from build123d import *

# Parameters (mm, degrees)
BOSS_EXTRUDE1_DEPTH      = 52.5
BOSS_EXTRUDE1_DEPTH_BACK = 52.5
BOSS_EXTRUDE2_DEPTH      = 13
BOSS_EXTRUDE3_DEPTH      = 13
CUT_EXTRUDE1_DEPTH       = 65.5
CUT_EXTRUDE1_DEPTH_BACK  = 65.5
CUT_EXTRUDE2_DEPTH       = 29
CUT_EXTRUDE2_DEPTH_BACK  = 29
CUT_EXTRUDE3_DEPTH       = 29
CUT_EXTRUDE3_DEPTH_BACK  = 29
SKETCH7_R                = 2.6
CUT_EXTRUDE4_DEPTH       = 1
SKETCH8_R                = 2.6
CUT_EXTRUDE5_DEPTH       = 1
CUT_EXTRUDE6_START       = 1
SKETCH9_R                = 2.6
CUT_EXTRUDE6_DEPTH       = 1
CUT_EXTRUDE7_START       = 1
SKETCH10_R               = 2.6
CUT_EXTRUDE7_DEPTH       = 1
CUT_EXTRUDE8_DEPTH       = 35
CUT_EXTRUDE9_DEPTH       = 35


with BuildPart() as part:
    # Sketch1 → Boss-Extrude1 (new, two sides: drawn at the far end of the back side and taken through both)
    with BuildSketch(Plane(origin=(0, 0, 0), x_dir=(0, 0, -1), z_dir=(1, 0, 0)).offset(-BOSS_EXTRUDE1_DEPTH_BACK)):
        with BuildLine():
            Line((-30, 33), (-30, 27))
            Line((-30, 27), (-29.5, 26.5))
            Line((-29.5, 26.5), (-29.5, 2))
            ThreePointArc((-29.5, 2), (-28.914213562, 0.585786438), (-27.5, 0))
            Line((-27.5, 0), (27.5, 0))
            ThreePointArc((27.5, 0), (28.914213562, 0.585786438), (29.5, 2))
            Line((29.5, 2), (29.5, 26.5))
            Line((29.5, 26.5), (30, 27))
            Line((30, 27), (30, 33))
            Line((30, 33), (28, 35))
            Line((28, 35), (10, 35))
            Line((10, 35), (9.5, 34.5))
            Line((9.5, 34.5), (-9.5, 34.5))
            Line((-9.5, 34.5), (-10, 35))
            Line((-10, 35), (-28, 35))
            Line((-28, 35), (-30, 33))
        make_face()
    extrude(amount=BOSS_EXTRUDE1_DEPTH + BOSS_EXTRUDE1_DEPTH_BACK)

    # Sketch2 → Boss-Extrude2 (add)
    with BuildSketch(Plane(origin=(-65.5, 0, 0), x_dir=(0, 0, -1), z_dir=(1, 0, 0))):
        Polygon((-29, 2), (-27, 0), (27, 0), (29, 2), (29, 32.5), (27.5, 34), (-27.5, 34), (-29, 32.5), align=None)
    extrude(amount=BOSS_EXTRUDE2_DEPTH)

    # Sketch3 → Boss-Extrude3 (add)
    with BuildSketch(Plane(origin=(65.5, 0, 0), x_dir=(0, 0, -1), z_dir=(1, 0, 0))):
        Polygon((-29, 2), (-27, 0), (27, 0), (29, 2), (29, 32.5), (27.5, 34), (-27.5, 34), (-29, 32.5), align=None)
    extrude(amount=-BOSS_EXTRUDE3_DEPTH)

    # Sketch4 → Cut-Extrude1 (cut, two sides: drawn at the far end of the back side and taken through both)
    with BuildSketch(Plane(origin=(0, 0, 0), x_dir=(0, 0, -1), z_dir=(1, 0, 0)).offset(-CUT_EXTRUDE1_DEPTH_BACK)):
        with BuildLine():
            Line((-14, 13.148439), (-14, 11.35158))
            ThreePointArc((-14, 11.35158), (-13.885407957, 11.031881418), (-13.592386868, 10.860192277))
            ThreePointArc((-13.592386868, 10.860192277), (-12.229021504, 10.099202354), (-11.602627372, 8.66899217))
            ThreePointArc((-11.602627372, 8.66899217), (-11.559004129, 8.501191683), (-11.458152391, 8.360163609))
            Line((-11.458152391, 8.360163609), (-11.005017, 7.906991))
            ThreePointArc((-11.005017, 7.906991), (-10.852063473, 7.680418582), (-10.800003, 7.412054))
            Line((-10.800003, 7.412054), (-10.800003, 3.490777069))
            ThreePointArc((-10.800003, 3.490777069), (-10.853443426, 3.222114259), (-11.005628687, 2.994352913))
            Line((-11.005628687, 2.994352913), (-13.795574427, 0.204407575))
            ThreePointArc((-13.795574427, 0.204407575), (-13.946871354, -0.022023954), (-14, -0.289118216))
            Line((-14, -0.289118216), (-14, -5.5))
            Line((-14, -5.5), (-12.5, -7))
            Line((-12.5, -7), (-5.0000003, -7))
            Line((-5.0000003, -7), (-4.499985, -6.50000763))
            Line((-4.499985, -6.50000763), (4.499985, -6.50000763))
            Line((4.499985, -6.50000763), (5.0000003, -7))
            Line((5.0000003, -7), (12.5, -7))
            Line((12.5, -7), (14, -5.5))
            Line((14, -5.5), (14, -0.289118216))
            ThreePointArc((14, -0.289118216), (13.946871354, -0.022023954), (13.795574427, 0.204407575))
            Line((13.795574427, 0.204407575), (11.005628687, 2.994352913))
            ThreePointArc((11.005628687, 2.994352913), (10.853443426, 3.222114259), (10.800003, 3.490777069))
            Line((10.800003, 3.490777069), (10.800003, 7.412054))
            ThreePointArc((10.800003, 7.412054), (10.852063473, 7.680418582), (11.005017, 7.906991))
            Line((11.005017, 7.906991), (11.458152391, 8.360163609))
            ThreePointArc((11.458152391, 8.360163609), (11.559004129, 8.501191683), (11.602627372, 8.66899217))
            ThreePointArc((11.602627372, 8.66899217), (12.229021504, 10.099202354), (13.592386868, 10.860192277))
            ThreePointArc((13.592386868, 10.860192277), (13.885407957, 11.031881418), (14, 11.35158))
            Line((14, 11.35158), (14, 13.148439))
            ThreePointArc((14, 13.148439), (13.886532321, 13.469052961), (13.5924176, 13.639829881))
            ThreePointArc((13.5924176, 13.639829881), (12.312672018, 14.314596081), (11.635789981, 15.593223817))
            ThreePointArc((11.635789981, 15.593223817), (11.466717508, 15.887148006), (11.146965482, 16))
            Line((11.146965482, 16), (-11.146965482, 16))
            ThreePointArc((-11.146965482, 16), (-11.466717508, 15.887148006), (-11.635789981, 15.593223817))
            ThreePointArc((-11.635789981, 15.593223817), (-12.312672018, 14.314596081), (-13.5924176, 13.639829881))
            ThreePointArc((-13.5924176, 13.639829881), (-13.886532321, 13.469052961), (-14, 13.148439))
        make_face()
    extrude(amount=CUT_EXTRUDE1_DEPTH + CUT_EXTRUDE1_DEPTH_BACK, mode=Mode.SUBTRACT)

    # Sketch5 → Cut-Extrude2 (cut, two sides: drawn at the far end of the back side and taken through both)
    with BuildSketch(Plane.XY.offset(-CUT_EXTRUDE2_DEPTH_BACK)):
        Polygon((-65.5, 33.5), (-65, 34), (-65.5, 34), align=None)
    extrude(amount=CUT_EXTRUDE2_DEPTH + CUT_EXTRUDE2_DEPTH_BACK, mode=Mode.SUBTRACT)

    # Sketch6 → Cut-Extrude3 (cut, two sides: drawn at the far end of the back side and taken through both)
    with BuildSketch(Plane.XY.offset(-CUT_EXTRUDE3_DEPTH_BACK)):
        Polygon((65, 34), (65.5, 33.5), (65.5, 34), align=None)
    extrude(amount=CUT_EXTRUDE3_DEPTH + CUT_EXTRUDE3_DEPTH_BACK, mode=Mode.SUBTRACT)

    # Sketch7 → Cut-Extrude4 (cut)
    with BuildSketch(Plane.XY.offset(29)):
        with Locations((58.3, 29)):
            Circle(SKETCH7_R)
    extrude(amount=-CUT_EXTRUDE4_DEPTH, mode=Mode.SUBTRACT)

    # Sketch8 → Cut-Extrude5 (cut)
    with BuildSketch(Plane.XY.offset(29)):
        with Locations((-58.3, 29)):
            Circle(SKETCH8_R)
    extrude(amount=-CUT_EXTRUDE5_DEPTH, mode=Mode.SUBTRACT)

    # Sketch9 → Cut-Extrude6 (cut)
    with BuildSketch(Plane.XY.offset(-29).offset(CUT_EXTRUDE6_START)):
        with Locations((58.3, 29)):
            Circle(SKETCH9_R)
    extrude(amount=-CUT_EXTRUDE6_DEPTH, mode=Mode.SUBTRACT)

    # Sketch10 → Cut-Extrude7 (cut)
    with BuildSketch(Plane.XY.offset(-29).offset(CUT_EXTRUDE7_START)):
        with Locations((-58.3, 29)):
            Circle(SKETCH10_R)
    extrude(amount=-CUT_EXTRUDE7_DEPTH, mode=Mode.SUBTRACT)

    # Sketch11 → Cut-Revolve1 (revolve, cut)
    with BuildSketch(Plane.XY, mode=Mode.PRIVATE) as cut_revolve1_sk:
        Polygon((-65.5, 27), (-65.5, 30), (-64.9585, 29.4585), (-59.5, 29.4585), (-58.080584363, 27), align=None)
    revolve(cut_revolve1_sk.sketch.rotate(Axis((-58.080584363, 27, 0), (-1, 0, 0)), 270), axis=Axis((-58.080584363, 27, 0), (-1, 0, 0)), mode=Mode.SUBTRACT)

    # Sketch12 → Cut-Revolve2 (revolve, cut)
    with BuildSketch(Plane.XY, mode=Mode.PRIVATE) as cut_revolve2_sk:
        Polygon((58.080584363, 27), (59.5, 29.4585), (64.9585, 29.4585), (65.5, 30), (65.5, 27), align=None)
    revolve(cut_revolve2_sk.sketch.rotate(Axis((65.5, 27, 0), (-1, 0, 0)), 270), axis=Axis((65.5, 27, 0), (-1, 0, 0)), mode=Mode.SUBTRACT)

    # Sketch13 → Cut-Revolve3 (revolve, cut)
    with BuildSketch(Plane.XY.offset(20), mode=Mode.PRIVATE) as cut_revolve3_sk:
        Polygon((-30, 35), (-26, 35), (-26.6765, 34.3235), (-26.6765, 25.4), (-30, 23.48117638), align=None)
    revolve(cut_revolve3_sk.sketch.rotate(Axis((-30, 23.48117638, 20), (0, 1, 0)), 270), axis=Axis((-30, 23.48117638, 20), (0, 1, 0)), mode=Mode.SUBTRACT)

    # Sketch14 → Cut-Revolve4 (revolve, cut)
    with BuildSketch(Plane.XY.offset(20), mode=Mode.PRIVATE) as cut_revolve4_sk:
        Polygon((30, 35), (34, 35), (33.3235, 34.3235), (33.3235, 25.4), (30, 23.48117638), align=None)
    revolve(cut_revolve4_sk.sketch.rotate(Axis((30, 23.48117638, 20), (0, 1, 0)), 270), axis=Axis((30, 23.48117638, 20), (0, 1, 0)), mode=Mode.SUBTRACT)

    # Sketch15 → Cut-Revolve5 (revolve, cut)
    with BuildSketch(Plane.XY.offset(-20), mode=Mode.PRIVATE) as cut_revolve5_sk:
        Polygon((-30, 35), (-26, 35), (-26.6765, 34.3235), (-26.6765, 25.4), (-30, 23.48117638), align=None)
    revolve(cut_revolve5_sk.sketch.rotate(Axis((-30, 23.48117638, -20), (0, 1, 0)), 270), axis=Axis((-30, 23.48117638, -20), (0, 1, 0)), mode=Mode.SUBTRACT)

    # Sketch16 → Cut-Revolve6 (revolve, cut)
    with BuildSketch(Plane.XY.offset(-20), mode=Mode.PRIVATE) as cut_revolve6_sk:
        Polygon((30, 35), (34, 35), (33.3235, 34.3235), (33.3235, 25.4), (30, 23.48117638), align=None)
    revolve(cut_revolve6_sk.sketch.rotate(Axis((30, 23.48117638, -20), (0, 1, 0)), 270), axis=Axis((30, 23.48117638, -20), (0, 1, 0)), mode=Mode.SUBTRACT)

    # Sketch17 → Cut-Extrude8 (cut)
    with BuildSketch(Plane(origin=(0, 0, 0), x_dir=(1, 0, 0), z_dir=(0, 1, 0))):
        Polygon((-130.5, 29.5), (-130.5, -29.5), (-65, -29.5), (-65, -29), (-65.5, -28.5), (-65.5, -29), (-130, -29), (-130, 29), (-65.5, 29), (-65.5, 28.5), (-65, 29), (-65, 29.5), align=None)
    extrude(amount=CUT_EXTRUDE8_DEPTH, mode=Mode.SUBTRACT)

    # Sketch18 → Cut-Extrude9 (cut)
    with BuildSketch(Plane(origin=(0, 0, 0), x_dir=(1, 0, 0), z_dir=(0, 1, 0))):
        Polygon((65, -29), (65, -29.5), (130.5, -29.5), (130.5, 29.5), (65, 29.5), (65, 29), (65.5, 28.5), (65.5, 29), (130, 29), (130, -29), (65.5, -29), (65.5, -28.5), align=None)
    extrude(amount=CUT_EXTRUDE9_DEPTH, mode=Mode.SUBTRACT)


solid = part.part
Geometry check sheet. Reference: the model listing, model coordinates, mm. A direction names the side the tool comes from. Round coordinates to 2 decimals unless told otherwise and drop trailing zeros. Loops run counter-clockwise (first coordinate to the right, second up) from the corner with the lowest first, then second, coordinate; pieces in that order, holes last. Notation, with made-up numbers: (21, 86.25) - (42, 86.25) arc R16 cw to (42, 107.25) - close; hole circle Ø4 at (31, 13). An arc over 180 degrees is marked (long way). One line per question, with ' | ' between items. Start each with the question number.
1. Cross-section at A-A on z = -7. Record the cut outline in (x, y), then the cut area to 3 significant figures.
2. Scan lines: line 1 (X direction, y = 31.5, z = -20); line 2 (Y direction, x = 62.45, z = 0); line 3 (Z direction, x = -55, y = 4.5). Record each from-to range of solid material in increasing order. Write a range as [from, to].
3. Depth check by flat-ended pin: pin 1 (3 mm diameter, centred on y = 27, z = 0, fed in from +X); pin 2 (3 mm diameter, centred on x = 42.5, z = -6, fed in from +Y); pin 3 (1.2 mm diameter, centred on x = -2, y = 4.5, fed in from -Z). Enter the tip coordinate at first touch or a pass-through.
4. Draft check along Y on faces 6 (the face through (-1, 30, 30)), 7 (the face through (58.327, 27.423, -0.056)), 8 (the face through (30.53, 23.79, 19.93)). Enter one of: released by +Y, released by -Y, zero draft, split by the parting line, or undercut.
5. Tool access check on faces 1 (the face through (-1, 34.5, 0)), 2 (the face through (62.3, 24.8, 1.1)), 3 (the face through (32.8, 29.8, 21.79)), 4 (the face through (-1, 0, -21)), 5 (the face through (-58, 29, -28)). Record the directions out of +Z, -Z, +X, -X, +Y, -Y that give a thin tool (end or side, any length) a straight path to the whole face; none if there is none.
Taken from the geometry:
1) outline: (-65.5, 16) - (65.5, 16) - (65.5, 33.5) - (65, 34) - (52.5, 34) - (52.5, 34.5) - (-52.5, 34.5) - (-52.5, 34) - (-65, 34) - (-65.5, 33.5) - close | area: 2,410 mm²
2) line 1: [-65.5, -33.32], [-26.68, 26.68], [33.32, 65.5] | line 2: [16, 24.54], [29.46, 34] | line 3: [-29, -10.8], [10.8, 29]
3) pin 1: x = 58.95 | pin 2: y = 34.5 | pin 3: z = -29.5
4) face 6: zero draft | face 7: undercut | face 8: released by +Y
5) face 1: +X, -X, +Y | face 2: +X | face 3: +Y | face 4: +Z, -Z, +X, -X, -Y | face 5: -Z
